The listing builds one solid part. Answer for the finished solid, in the listing's coordinates (mm). A direction names the side the tool comes from. Give positions to 0.01 mm unless a question says otherwise; leave off trailing zeros. Write each loop counter-clockwise with the first axis right and the second up, starting at its lowest first coordinate (ties: lowest second). Pieces come first, ordered by that corner, then holes. Notation, with made-up numbers: (54, 11) - (103, 11) arc R8 cw to (103, 25) - close; hole circle Ø2 at (40.25, -24). An arc over 180 degrees is marked (long way). Return JSON: item names as keys, results as strings.
from build123d import *

# Parameters (mm, degrees)
BOSS_EXTRUDE1_DEPTH = 228.6
SKETCH5_R           = 3.175
CUT_EXTRUDE1_DEPTH  = 229.99128374
SKETCH5_4_R         = 4.7625
CUT_EXTRUDE2_DEPTH  = 6.35


with BuildPart() as part:
    # Sketch1 → Boss-Extrude1 (new body)
    with BuildSketch(Plane(origin=(0, 0, 0), x_dir=(0, 0, -1), z_dir=(1, 0, 0))):
        Polygon((9.525, -0.254), (9.525, 3.048), (5.842, 3.048), (8.89, 8.327290861), (8.89, 9.398), (6.604, 9.398), (6.604, 9.144), (0, 9.144), (0, 0), (6.985, 0), (6.985, -0.254), align=None)
    boss_extrude1 = extrude(amount=BOSS_EXTRUDE1_DEPTH)

    # Mirror1: Boss-Extrude1 across plane
    add(boss_extrude1.mirror(Plane.XY))

    # Sketch4 → Tap Drill for _8-32 Tap2 (revolve, cut)
    with BuildSketch(Plane.ZX.offset(4.826)):
        Polygon((0, 0), (0, 13.737806461), (1.7272, 12.7), (1.7272, 0.635), (2.3622, 0), align=None)
    tap_drill_for_8_32_tap2 = revolve(axis=Axis((-6.35, 4.826, 0), (1, 0, 0)), mode=Mode.SUBTRACT)

    # Mirror2: Tap Drill for _8-32 Tap2 across plane
    add(tap_drill_for_8_32_tap2.mirror(Plane.ZY.offset(-114.3)), mode=Mode.SUBTRACT)

    # Sketch5 → Cut-Extrude1 (cut, through all)
    with BuildSketch(Plane(origin=(0, 9.144, 0), x_dir=(1, 0, 0), z_dir=(0, 1, 0))):
        with Locations(Location((25.4, 0, 0), (0, 0, 270))):
            Circle(SKETCH5_R)
        with Locations(Location((101.6, 0, 0), (0, 0, 270))):
            Circle(SKETCH5_R)
        with Locations(Location((127, 0, 0), (0, 0, 270))):
            Circle(SKETCH5_R)
        with Locations(Location((203.2, 0, 0), (0, 0, 270))):
            Circle(SKETCH5_R)
        with BuildLine():
            Line((50.8, 3.175), (76.2, 3.175))
            ThreePointArc((76.2, 3.175), (79.375, 0), (76.2, -3.175))
            Line((76.2, -3.175), (50.8, -3.175))
            ThreePointArc((50.8, -3.175), (47.625, 0), (50.8, 3.175))
        make_face()
        with BuildLine():
            Line((152.4, 3.175), (177.8, 3.175))
            ThreePointArc((177.8, 3.175), (180.975, 0), (177.8, -3.175))
            Line((177.8, -3.175), (152.4, -3.175))
            ThreePointArc((152.4, -3.175), (149.225, 0), (152.4, 3.175))
        make_face()
    extrude(amount=-CUT_EXTRUDE1_DEPTH, mode=Mode.SUBTRACT)

    # Sketch5_4 → Cut-Extrude2 (cut)
    with BuildSketch(Plane(origin=(0, 9.144, 0), x_dir=(1, 0, 0), z_dir=(0, 1, 0))):
        with Locations(Location((25.4, 0, 0), (0, 0, 270))):
            Circle(SKETCH5_4_R)
        with Locations(Location((101.6, 0, 0), (0, 0, 270))):
            Circle(SKETCH5_4_R)
        with Locations(Location((127, 0, 0), (0, 0, 270))):
            Circle(SKETCH5_4_R)
        with Locations(Location((203.2, 0, 0), (0, 0, 270))):
            Circle(SKETCH5_4_R)
        with BuildLine():
            Line((50.8, 4.7625), (76.2, 4.7625))
            ThreePointArc((76.2, 4.7625), (80.9625, 0), (76.2, -4.7625))
            Line((76.2, -4.7625), (50.8, -4.7625))
            ThreePointArc((50.8, -4.7625), (46.0375, 0), (50.8, 4.7625))
        make_face()
        with BuildLine():
            Line((152.4, 4.7625), (177.8, 4.7625))
            ThreePointArc((177.8, 4.7625), (182.5625, 0), (177.8, -4.7625))
            Line((177.8, -4.7625), (152.4, -4.7625))
            ThreePointArc((152.4, -4.7625), (147.6375, 0), (152.4, 4.7625))
        make_face()
    extrude(amount=-CUT_EXTRUDE2_DEPTH, mode=Mode.SUBTRACT)


solid = part.part
Item 1: A cutting plane is placed at B-B on x = 137. Determine the outline of the cut face in (y, z) (3 decimals), then the cut area to 3 significant figures.
Answer below:
{"outline": "(-0.254, -9.525) - (3.048, -9.525) - (3.048, -5.842) - (8.327, -8.89) - (9.398, -8.89) - (9.398, -6.604) - (9.144, -6.604) - (9.144, 6.604) - (9.398, 6.604) - (9.398, 8.89) - (8.327, 8.89) - (3.048, 5.842) - (3.048, 9.525) - (-0.254, 9.525) - (-0.254, 6.985) - (0, 6.985) - (0, -6.985) - (-0.254, -6.985) - close", "area": "153 mm²"}
Item 2: The mould has two halves that part along X. Classify faces 1 (the face through (113, 9.144, 0)), 2 (the face through (215.04, 5.09, 0.14)), 3 (the face through (64, 6, 4.762)): +X half, -X half, draft (parallel to the pull), parting line (faces both ways), or undercut.
Answer below:
{"face 1": "draft", "face 2": "+X half", "face 3": "undercut"}
Item 3: For faces 4 (the face through (222.017, 3.113, -0.225)), 5 (the face through (80.96, 6.01, -0.1)), 6 (the face through (13.56, 5.09, 0.14)), determine the directions among +Z, -Z, +X, -X, +Y, -Y from which every point of the face is accessible in a straight line to the end or side of a thin tool.
Answer below:
{"face 4": "+X", "face 5": "+Y", "face 6": "-X"}
Item 4: Consider L1, parallel to Y at x = 206, z = 2; L2, parallel to Y at x = 39.5, z = 5.75; L3, parallel to Z at x = 203.2, y = 1.9 (3 decimals). Determine where each line is inside the solid, lowest interval first.
Answer below:
{"L1": "y = 0 to 2.79", "L2": "y = 0 to 9.14", "L3": "z = -9.525 to -3.175, 3.175 to 9.525"}
Item 5: Flat-ended cylindrical pins translate along their axes: P1, Ø7.5, axis at x = 202.5, z = 1, coming from the +Y side; P2, Ø1.9, axis at x = 165.5, y = 4.5, coming from the +Z side; P3, Ø4.5, axis at y = 4.826, z = 0, coming from the -X side. Find the tip coordinate at first contact, or state that the pin passes through.
Answer below:
{"P1": "stops at y = 9.14", "P2": "stops at z = 7.23", "P3": "stops at x = 0.11"}
